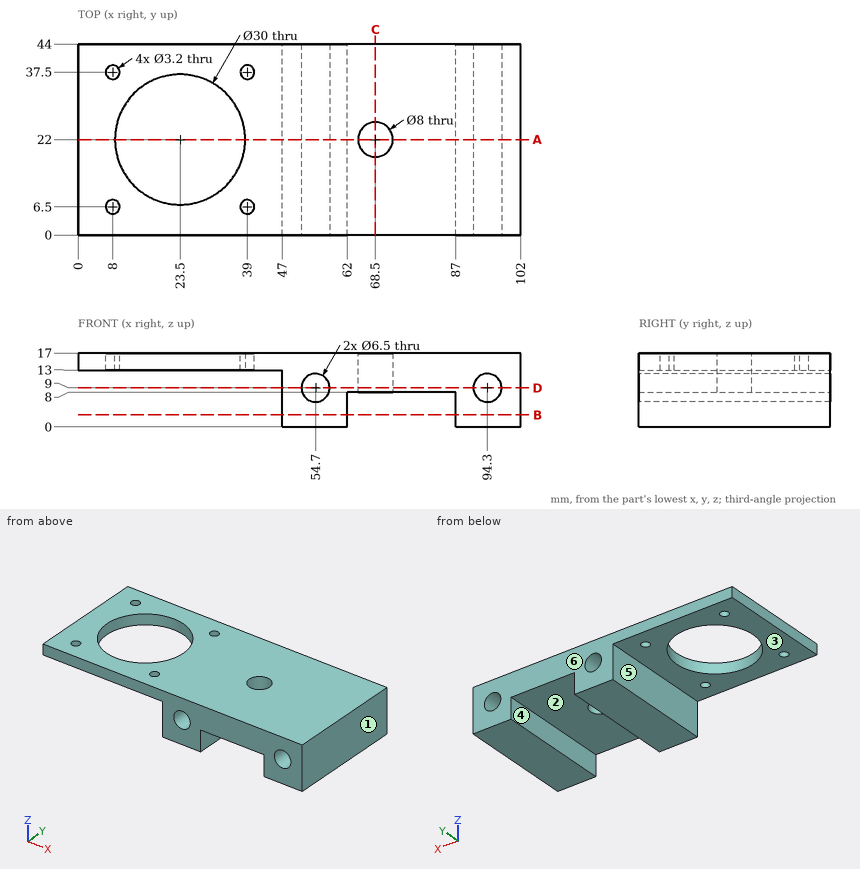
For this review, use the dimensioned drawing (mm, ordinates from the lowest corner) and the shaded views. A direction names the side the tool comes from. Coordinates: 2 decimals unless noted, no trailing zeros. Loops run counter-clockwise (first coordinate to the right, second up) from the corner with the lowest first, then second, coordinate; pieces in that order, holes last.
1. Add section B-B, the plane z = 2.75. Give the boundary of the cut face in (x, y), then the cut area to 3 significant figures.
2. For the marked faces 1, 2 and 3, list the 3-axis set-ups (+Z, -Z, +X, -X, +Y, -Y) from which the entire face can be reached by the end or side of a thin tool; tool diameter is ignored.
3. Mouldability with a two-part tool opening along X and no side actions: class the marked faces 4, 5 and 6 as +X half, -X half, draft (parallel to the pull), parting line (faces both ways), or undercut.
4. Add section C-C, the plane x = 68.5. Give the boundary of the cut face in (y, z), then the cut area to 3 significant figures.
5. For line 1 (X direction, y = 37.5, z = 15.65); line 2 (X direction, y = 13, z = 9); line 3 (X direction, y = 39, z = 1), list the stretches that pass through material, from the lowest coordinate up.
6. Insertion check: P1, Ø4, axis at y = 21, z = 4, coming from the -X side; P2, Ø6, axis at x = 80.5, y = 6, coming from the -Z side; P3, Ø4, axis at x = 8, y = 6.5, coming from the -Z side. Each pin has a flat end and moves straight along its axis. Give the tip position at first contact, or say it passes through.
7. Add section D-D, the plane z = 9. Give the boundary of the cut face in (x, y).
8. Add section A-A, the plane y = 22. Give the boundary of the cut face in (x, z), then the cut area to 3 significant figures.
Result:
1. outline: (47, 0) - (62, 0) - (62, 44) - (47, 44) - close; (87, 0) - (102, 0) - (102, 44) - (87, 44) - close
1. area: 1,320 mm2
2. face 1: +Z, -Z, +X, +Y, -Y
2. face 2: -Z, +Y, -Y
2. face 3: -Z, -X, +Y, -Y
3. face 4: undercut
3. face 5: -X half
3. face 6: draft
4. outline: (0, 8) - (18, 8) - (18, 17) - (0, 17) - close; (26, 8) - (44, 8) - (44, 17) - (26, 17) - close
4. area: 324 mm2
5. line 1: x = 0 to 6.4, 9.6 to 37.4, 40.6 to 102
5. line 2: x = 47 to 51.45, 57.95 to 91.05, 97.55 to 102
5. line 3: x = 47 to 62, 87 to 102
6. P1: stops at x = 47
6. P2: stops at z = 8
6. P3: stops at z = 13
7. outline: (47, 0) - (51.45, 0) - (51.45, 44) - (47, 44) - close; (57.95, 0) - (91.05, 0) - (91.05, 44) - (57.95, 44) - close; (97.55, 0) - (102, 0) - (102, 44) - (97.55, 44) - close; hole circle Ø8 at (68.5, 22)
8. outline: (0, 13) - (8.5, 13) - (8.5, 17) - (0, 17) - close; (38.5, 13) - (47, 13) - (47, 0) - (62, 0) - (62, 8) - (64.5, 8) - (64.5, 17) - (38.5, 17) - close; (72.5, 8) - (87, 8) - (87, 0) - (102, 0) - (102, 17) - (72.5, 17) - close; hole circle Ø6.5 at (54.7, 9); hole circle Ø6.5 at (94.3, 9)
8. area: 665 mm2
